Design review of the part built by this model. Coordinates are the model's own, in mm. Round coordinates to 2 decimals unless told otherwise and drop trailing zeros. Order: outer loops, then holes, each group sorted by start corner. A loop starts at its lowest first (then second) coordinate and runs counter-clockwise, first axis right, second up. Notation, with made-up numbers: M 4.25,89.5 L 33.25,89.5 A18 ccw 33.25,120.5 Z; hole C -1,86.5 d4. An arc over 180 degrees is marked long. Use a Markdown table: item, result. Add a question column.
(1) Take a section at C-C (z = 1.05). Write out the cut boundary in (x, y).
(2) To check wall thickness, follow probe 1 along X at (y, z) = (-1, 1); probe 2 along X at (y, z) = (1.75, 2.9); probe 3 along Y at (x, z) = (2.25, 2.85). State the ranges of each line that lie inside material, in increasing order. Write a range as from..to.
(3) Take a section at A-A (x = -1.5). Write out the cut boundary in (y, z), then the cut area to 3 significant figures.
(4) Take a section at B-B (y = 0). Write out the cut boundary in (x, z), then the cut area to 3 significant figures.
(5) The part is to be moulded in two halves that separate along Y. For faces 1 (the face through (3.352, 2.183, 1.479)), 2 (the face through (3.567, -1.811, 1.479)), 3 (the face through (-0.54, -2.44, 1.52)), say which applies: released by +Y, released by -Y, zero draft, split by the parting line, or undercut.
(6) For pin 1 (1 mm diameter, centred on y = 2.5, z = 0.5, fed in from +X), flat-tipped, find the tip position at first contact; note if it passes through.
```python
from build123d import *

# Parameters (mm, degrees)
EXTRUDE_1_DEPTH     = 3
CUT_EXTRUDE_1_REACH = 5
SKETCH_2_R          = 2.5


with BuildPart() as part:
    # 草圖1 → 填料-伸長1 (new body)
    with BuildSketch(Plane.XY):
        Polygon((2.058046104, 4.134946138), (-2.551945347, 3.849793278), (-4.609991451, -0.285152861), (-2.058046104, -4.134946138), (2.551945347, -3.849793278), (4.609991451, 0.285152861), align=None)
    extrude(amount=EXTRUDE_1_DEPTH)

    # 草圖2 → 除料-伸長1 (cut, up to next)
    with BuildSketch(Plane.XY.offset(3), mode=Mode.PRIVATE) as cut_extrude_1_sk1:
        Circle(SKETCH_2_R)
    cut_extrude_1_tool1 = extrude(cut_extrude_1_sk1.sketch, amount=-CUT_EXTRUDE_1_REACH, mode=Mode.PRIVATE) & part.part
    add(cut_extrude_1_tool1.solids().sort_by_distance((0, 0, 3))[0], mode=Mode.SUBTRACT)


solid = part.part
```
Verdict:
| question | item | result |
|---|---|---|
| 1 | outline | M -4.61,-0.29 L -2.06,-4.13 L 2.55,-3.85 L 4.61,0.29 L 2.06,4.13 L -2.55,3.85 Z; hole C 0,0 d5 |
| 2 | probe 1 | x = -4.14..-2.29, 2.29..3.97 |
| 2 | probe 2 | x = -3.6..-1.79, 1.79..3.64 |
| 2 | probe 3 | y = -3.87..-1.09, 1.09..3.85 |
| 3 | outline | M -4.1,0 L -2,0 L -2,3 L -4.1,3 Z; M 2,0 L 3.91,0 L 3.91,3 L 2,3 Z |
| 3 | area | 12.0 mm^2 |
| 4 | outline | M -4.47,0 L -2.5,0 L -2.5,3 L -4.47,3 Z; M 2.5,0 L 4.47,0 L 4.47,3 L 2.5,3 Z |
| 4 | area | 11.8 mm^2 |
| 5 | face 1 | released by +Y |
| 5 | face 2 | released by -Y |
| 5 | face 3 | undercut |
| 6 | pin 1 | stops at x = 3.47 |
